```python
from build123d import *

# Parameters (mm, degrees)
SKETCH2_R           = 2
SKETCH2_R_2         = 7.5
FLANGE_DEPTH        = 8.5
SKETCH3_R           = 8.5
O_RING_SEAT_DEPTH   = 0.5
SKETCH8_R           = 18
CUT_EXTRUDE1_DEPTH  = 7
SKETCH5_R           = 1
OUTLET_DEPTH        = 38.739236876
BOSS_EXTRUDE2_REACH = 50.576
SKETCH6_R           = 3
SKETCH6_R_2         = 1
INLET_COUNT         = 2


with BuildPart() as part:
    # Sketch2 → Flange (new, symmetric)
    with BuildSketch(Plane(origin=(0, 0, 0), x_dir=(0, 0, -1), z_dir=(1, 0, 0))):
        with BuildLine():
            ThreePointArc((-14.142135624, 14.142135624), (-26, 0), (-14.142135624, -14.142135624))
            ThreePointArc((-14.142135624, -14.142135624), (0, -26), (14.142135624, -14.142135624))
            ThreePointArc((14.142135624, -14.142135624), (26, 0), (14.142135624, 14.142135624))
            ThreePointArc((14.142135624, 14.142135624), (0, 26), (-14.142135624, 14.142135624))
        make_face()
        with Locations((0, 23)):
            Circle(SKETCH2_R, mode=Mode.SUBTRACT)
        with Locations((23, 0)):
            Circle(SKETCH2_R, mode=Mode.SUBTRACT)
        with Locations((0, -23)):
            Circle(SKETCH2_R, mode=Mode.SUBTRACT)
        with Locations((-23, 0)):
            Circle(SKETCH2_R, mode=Mode.SUBTRACT)
        Circle(SKETCH2_R_2, mode=Mode.SUBTRACT)
    extrude(amount=FLANGE_DEPTH, both=True)

    # Sketch3 → O-Ring Seat (cut)
    with BuildSketch(Plane(origin=(8.5, 0, 0), x_dir=(0, 0, -1), z_dir=(1, 0, 0))):
        Circle(SKETCH3_R)
    o_ring_seat = extrude(amount=-O_RING_SEAT_DEPTH, mode=Mode.SUBTRACT)

    # Mirror1: O-Ring Seat across plane
    add(o_ring_seat.mirror(Plane(origin=(0, 0, 0), x_dir=(0, 0, 1), z_dir=(1, 0, 0))), mode=Mode.SUBTRACT)

    # Sketch8 → Cut-Extrude1 (cut, symmetric)
    with BuildSketch(Plane.ZY):
        Circle(SKETCH8_R)
    extrude(amount=CUT_EXTRUDE1_DEPTH, both=True, mode=Mode.SUBTRACT)

    # Sketch5 → Outlet (cut, through all)
    with BuildSketch(Plane(origin=(0, 0, 0), x_dir=(1, 0, 0), z_dir=(0, 1, 0))):
        with Locations(Location((0, 17, 0), (0, 0, 90))):
            Circle(SKETCH5_R)
    outlet = extrude(amount=OUTLET_DEPTH, mode=Mode.SUBTRACT)

    # Sketch6 → Boss-Extrude2 (add, up to next)
    with BuildSketch(Plane(origin=(0, 14.142135624, 0), x_dir=(1, 0, 0), z_dir=(0, 1, 0)), mode=Mode.PRIVATE) as boss_extrude2_sk1:
        with Locations((0, 17)):
            Circle(SKETCH6_R)
        with Locations(Location((0, 17, 0), (0, 0, 90))):
            Circle(SKETCH6_R_2, mode=Mode.SUBTRACT)
    boss_extrude2_tool1 = extrude(boss_extrude2_sk1.sketch, amount=-BOSS_EXTRUDE2_REACH, mode=Mode.PRIVATE) - part.part
    boss_extrude2 = boss_extrude2_tool1.solids().sort_by_distance((-2.915147, 14.142136, -17))[0]
    add(boss_extrude2)

    # Sketch9 → Revolve1 (revolve)
    with BuildSketch(Plane(origin=(0, 0, 0), x_dir=(0, 0, -1), z_dir=(1, 0, 0)), mode=Mode.PRIVATE) as revolve1_sk:
        Polygon((18, 14.142135624), (18, 21.142135624), (18.5, 21.142135624), (19, 19.142135624), (18.5, 19.142135624), (19, 17.142135624), (18.5, 17.142135624), (19, 15.142135624), (18.5, 15.142135624), (18.5, 14.142135624), align=None)
    revolve1 = revolve(revolve1_sk.sketch.rotate(Axis((0, 14.142135624, -17), (0, -1, 0)), 180), axis=Axis((0, 14.142135624, -17), (0, -1, 0)))

    # Inlet: Outlet, Boss-Extrude2, Revolve1 ×2 about axis
    inlet_axis = Axis((8, 0, 0), (1, 0, 0))
    add([outlet.rotate(inlet_axis, i * 360 / INLET_COUNT) for i in range(1, INLET_COUNT)], mode=Mode.SUBTRACT)
    add([boss_extrude2.rotate(inlet_axis, i * 360 / INLET_COUNT) for i in range(1, INLET_COUNT)])
    add([revolve1.rotate(inlet_axis, i * 360 / INLET_COUNT) for i in range(1, INLET_COUNT)])


solid = part.part
```
CAD build for the part. Positions are in the model's coordinates, mm. A direction names the side the tool comes from. Round coordinates to 2 decimals unless told otherwise and drop trailing zeros. Write each loop counter-clockwise with the first axis right and the second up, starting at its lowest first coordinate (ties: lowest second). Pieces come first, ordered by that corner, then holes.
Item 1: Drill centre lines: L1, parallel to X at y = 8.5, z = -6; L2, parallel to Y at x = 3, z = -7; L3, parallel to Z at x = -4.5, y = -2.5. Where is each one in solid material? Low to high.
Filled in:
L1: x = -8.5 to -7, 7 to 8.5
L2: y = -24.18 to -16.58, 16.58 to 24.18
L3: z = -25.78 to -17.83, 17.83 to 25.78
Item 2: Band-saw the part on B-B on y = 3. Write the cut outline in (x, z).
Filled in:
outline: (-8.5, -25.68) - (8.5, -25.68) - (8.5, -7.95) - (8, -7.95) - (8, -6.87) - (7, -6.87) - (7, -17.75) - (0.66, -17.75) arc R1 cw to (-0.66, -17.75) - (-7, -17.75) - (-7, -6.87) - (-8, -6.87) - (-8, -7.95) - (-8.5, -7.95) - close; (-8.5, 7.95) - (-8, 7.95) - (-8, 6.87) - (-7, 6.87) - (-7, 17.75) - (7, 17.75) - (7, 6.87) - (8, 6.87) - (8, 7.95) - (8.5, 7.95) - (8.5, 25.68) - (-8.5, 25.68) - close
Item 3: Band-saw the part on C-C on z = -23. Write the cut outline in (x, y).
Filled in:
outline: (-8.5, -8.78) - (8.5, -8.78) - (8.5, -2) - (-8.5, -2) - close; (-8.5, 2) - (8.5, 2) - (8.5, 8.78) - (-8.5, 8.78) - close
Item 4: Band-saw the part on A-A on x = 4. Write the cut outline in (y, z).
Filled in:
outline: (-14.14, -14.14) arc R14.36 ccw to (14.14, -14.14) arc R14.36 ccw to (14.14, 14.14) arc R14.36 ccw to (-14.14, 14.14) arc R14.36 ccw to start; hole circle Ø4 at (-23, 0); hole circle Ø36 at (0, 0); hole circle Ø4 at (0, -23); hole circle Ø4 at (0, 23); hole circle Ø4 at (23, 0)
Item 5: Drop flat-ended pins along their axis: pin 1 Ø4.5 at (x, z) = (-0.5, 16.5) entering from -Y; pin 2 Ø3 at (x, z) = (3, -3) entering from +Y; pin 3 Ø2.5 at (x, z) = (0, 17) entering from +Y; pin 4 Ø6.5 at (y, z) = (0, -23) entering from -X. Give the stop position or say it passes through.
Filled in:
pin 1: stops at y = -21.14
pin 2: stops at y = 25.92
pin 3: stops at y = 13.76
pin 4: stops at x = -8.5
Item 6: Tool access for faces 1 (the cylindrical face through (-8.254, 7.167, -4.57)), 2 (the flat face through (8, -8, 0)), 3 (the conical face through (0.999, 20.573, -18.303)), 4 (the cylindrical face through (0, -21, 0)), 5 (the flat face through (1.3, 14.142, -15.8)): list every direction of +Z, -Z, +X, -X, +Y, -Y with a clear straight run to the whole face (end or side of a thin tool).
Filled in:
face 1: -X
face 2: +X
face 3: +Y
face 4: +X, -X
face 5: none
